Source: CAD feature listing. Evaluate the final solid. Frame: model axes, mm. A direction names the side the tool comes from. Round coordinates to 2 decimals unless told otherwise and drop trailing zeros. Write each loop counter-clockwise with the first axis right and the second up, starting at its lowest first coordinate (ties: lowest second). Pieces come first, ordered by that corner, then holes. Notation, with made-up numbers: M 85,34 L 139,34 A14 cw 139,49 Z; hole C 25,-35 d8. An arc over 180 degrees is marked long. Answer in a Markdown table with one row per item.
from build123d import *

# Parameters (mm, degrees)
SKETCH1_W                                           = 30.2
SKETCH1_H                                           = 55.8
BOSS_EXTRUDE1_DEPTH                                 = 8.35
CBORE_FOR_M4_HEX_SOCKET_HEAD_CAP_SCREW1_D           = 4.5
CBORE_FOR_M4_HEX_SOCKET_HEAD_CAP_SCREW1_CBORE_D     = 8
CBORE_FOR_M4_HEX_SOCKET_HEAD_CAP_SCREW1_CBORE_DEPTH = 4.4
BOSS_EXTRUDE2_START                                 = -15
SKETCH4_R                                           = 6
BOSS_EXTRUDE2_DEPTH                                 = 43.6


with BuildPart() as part:
    # Sketch1 → Boss-Extrude1 (new body, symmetric)
    with BuildSketch(Plane.XY):
        Rectangle(SKETCH1_W, SKETCH1_H)
    extrude(amount=BOSS_EXTRUDE1_DEPTH, both=True)

    # CBORE for M4 Hex Socket Head Cap Screw1 (through all)
    with Locations(Plane.XY.offset(8.35)):
        with Locations((-10, 12.9), (10, 12.9)):
            CounterBoreHole(CBORE_FOR_M4_HEX_SOCKET_HEAD_CAP_SCREW1_D / 2, CBORE_FOR_M4_HEX_SOCKET_HEAD_CAP_SCREW1_CBORE_D / 2, CBORE_FOR_M4_HEX_SOCKET_HEAD_CAP_SCREW1_CBORE_DEPTH)

    # Sketch4 → Boss-Extrude2 (add)
    with BuildSketch(Plane(origin=(0, 27.9, 0), x_dir=(1, 0, 0), z_dir=(0, 1, 0)).offset(BOSS_EXTRUDE2_START)):
        Circle(SKETCH4_R)
    extrude(amount=BOSS_EXTRUDE2_DEPTH)


solid = part.part
Q1. Access query for faces 4 (the cylindrical face through (-12.95, 15.6, 6.18)), 5 (the cylindrical face through (-6, 42, 0)), 6 (the cylindrical face through (-8.34, 14.42, -2.29)). Directions: +Z, -Z, +X, -X, +Y, -Y. A direction counts if a zero-diameter tool reaches every point of the face in a straight line with its end or side. Return the directions, or none.
Solutions:
| item | result |
|---|---|
| face 4 | +Z |
| face 5 | +Y |
| face 6 | +Z, -Z |
Q2. Contact query for flat-ended pins moving along their axis: pin 1 Ø4 at (x, y) = (-9, 12.5) entering from +Z; pin 2 Ø8 at (y, z) = (46, 4.5) entering from +X; pin 3 Ø4 at (x, z) = (8.5, -3.5) entering from +Y; pin 4 Ø2.5 at (x, y) = (10, 12.9) entering from +Z. Output: stop coordinate, or through.
Solutions:
| item | result |
|---|---|
| pin 1 | stops at z = 3.95 |
| pin 2 | stops at x = 5.98 |
| pin 3 | stops at y = 27.9 |
| pin 4 | passes through |
Q3. Section B-B (y = 12.9). Return loops of the section in (x, z).
Solutions:
| item | result |
|---|---|
| outline | M -15.1,-8.35 L -12.25,-8.35 L -12.25,3.95 L -14,3.95 L -14,8.35 L -15.1,8.35 Z; M -7.75,-8.35 L 7.75,-8.35 L 7.75,3.95 L 6,3.95 L 6,8.35 L -6,8.35 L -6,3.95 L -7.75,3.95 Z; M 12.25,-8.35 L 15.1,-8.35 L 15.1,8.35 L 14,8.35 L 14,3.95 L 12.25,3.95 Z |
Q4. Section A-A (x = 10). Return loops of the section in (y, z).
Solutions:
| item | result |
|---|---|
| outline | M -27.9,-8.35 L 10.65,-8.35 L 10.65,3.95 L 8.9,3.95 L 8.9,8.35 L -27.9,8.35 Z; M 15.15,-8.35 L 27.9,-8.35 L 27.9,8.35 L 16.9,8.35 L 16.9,3.95 L 15.15,3.95 Z |
Q5. Material intervals for probe 1 along Y at (x, z) = (-10, 4.9); probe 2 along Y at (x, z) = (-7.5, -3); probe 3 along Y at (x, z) = (-10, 0.25), sorted ascending.
Solutions:
| item | result |
|---|---|
| probe 1 | y = -27.9 to 8.9, 16.9 to 27.9 |
| probe 2 | y = -27.9 to 27.9 |
| probe 3 | y = -27.9 to 10.65, 15.15 to 27.9 |
Q6. Section D-D (x = 3). Return loops of the section in (y, z).
Solutions:
| item | result |
|---|---|
| outline | M -27.9,-8.35 L 27.9,-8.35 L 27.9,-5.2 L 56.5,-5.2 L 56.5,5.2 L 27.9,5.2 L 27.9,8.35 L -27.9,8.35 Z |
Q7. Pull-direction query (Y, two-part tool) for faces 1 (the cylindrical face through (7.05, 15.6, 6.18)), 2 (the flat face through (0, -27.9, 0)), 3 (the flat face through (-15.1, 0, 0)); classes: pulls with the +Y half, pulls with the -Y half, needs draft (parallel to the pull), parting line crosses it, or undercut.
Solutions:
| item | result |
|---|---|
| face 1 | undercut |
| face 2 | pulls with the -Y half |
| face 3 | needs draft |
Q8. Section C-C (z = 0). Return loops of the section in (x, y).
Solutions:
| item | result |
|---|---|
| outline | M -15.1,-27.9 L 15.1,-27.9 L 15.1,27.9 L 6,27.9 L 6,56.5 L -6,56.5 L -6,27.9 L -15.1,27.9 Z; hole C -10,12.9 d4.5; hole C 10,12.9 d4.5 |
